For this review, use the dimensioned drawing (mm, ordinates from the lowest corner) and the shaded views. Give positions to 0.01 mm unless a question says otherwise; leave off trailing zeros. Order: outer loops, then holes, each group sorted by start corner. A loop starts at its lowest first (then second) coordinate and runs counter-clockwise, first axis right, second up.
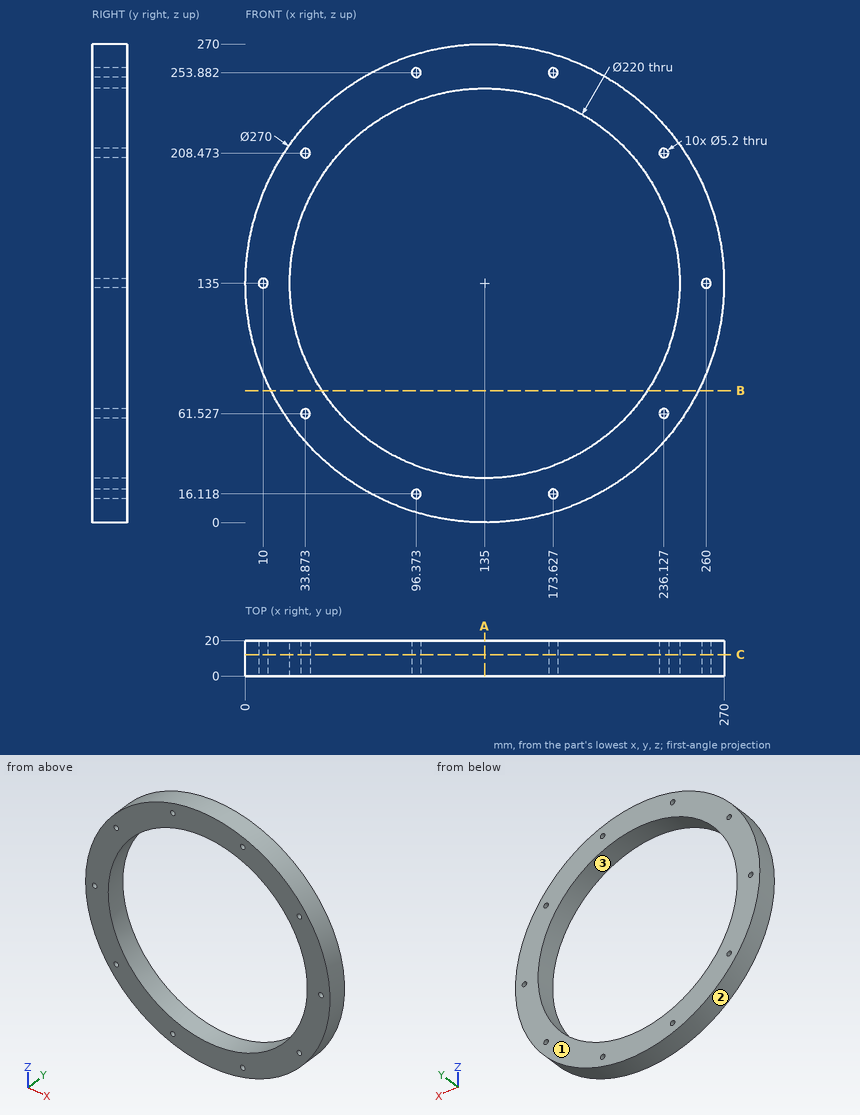
1. To check wall thickness, follow line 1 (X direction, y = 7.5, z = 137) (1 decimal); line 2 (Z direction, x = 236, y = 15.5) (1 decimal); line 3 (X direction, y = 18, z = 178). State the ranges of each line that lie inside material, in increasing order.
2. Take a section at C-C (y = 12). Count the separate pieces of the cut face and the enclosed holes in it, and give its area (3 significant figures).
3. Take a section at B-B (z = 74.5). Write out the cut boundary in (x, y).
4. Insertion check: pin 1 (2 mm diameter, centred on y = 4.5, z = 227.5, fed in from +X); pin 2 (10 mm diameter, centred on x = 215, y = 10, fed in from +Z). Each pin has a flat end and moves straight along its axis. Give the tip position at first contact, or say it passes through.
5. Take a section at A-A (x = 135). Write out the cut boundary in (y, z).
6. Draft analysis for pull direction X (two halves, no side actions). For the marked faces 1, 2 and 3, state which applies: pulls with the +X half, pulls with the -X half, needs draft (parallel to the pull), parting line crosses it, or undercut.
Answer:
1. line 1: x = 0 to 8.3, 11.7 to 25, 245 to 258.3, 261.7 to 270
1. line 2: z = 45.4 to 58.9, 64.1 to 91.4, 178.6 to 205.9, 211.1 to 224.6
1. line 3: x = 7.03 to 33.75, 236.25 to 262.97
2. separate pieces: 1
2. enclosed holes: 11
2. area: 19,000 mm2
3. outline: (14.32, 0) - (43.13, 0) - (43.13, 20) - (14.32, 20) - close; (226.87, 0) - (255.68, 0) - (255.68, 20) - (226.87, 20) - close
4. pin 1: stops at x = 234.26
4. pin 2: stops at z = 247.25
5. outline: (0, 0) - (20, 0) - (20, 25) - (0, 25) - close; (0, 245) - (20, 245) - (20, 270) - (0, 270) - close
6. face 1: needs draft
6. face 2: parting line crosses it
6. face 3: undercut
